Input: part model. Units: mm. Frame: model coordinates. Give positions to 0.01 mm unless a question says otherwise; leave off trailing zeros. Write each loop counter-clockwise with the first axis right and the second up, starting at its lowest first coordinate (ties: lowest second). Pieces come first, ordered by that corner, then holes. Notation, with made-up numbers: (76, -2) - (102, -2) arc R28 cw to (102, 21) - close; hole circle Ø7 at (8.25, 38.5). An arc over 180 degrees is marked (long way). Answer as CSV lines item,"result".
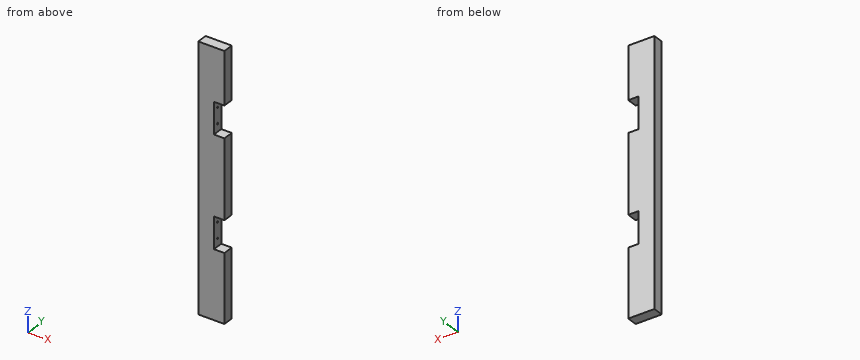
```python
from build123d import *

# Parameters (mm, degrees)
SKIZZE1_W                       = 50
SKIZZE1_H                       = 20
AUFSATZ_LINEAR_AUSTRAGEN1_DEPTH = 500
SKIZZE2_W                       = 20
SKIZZE2_H                       = 60
SCHNITT_LINEAR_AUSTRAGEN1_DEPTH = 502.023951523
SKIZZE3_R                       = 1.5
SCHNITT_LINEAR_AUSTRAGEN2_DEPTH = 20


with BuildPart() as part:
    # Skizze1 → Aufsatz-Linear austragen1 (new body)
    with BuildSketch(Plane.XY):
        Rectangle(SKIZZE1_W, SKIZZE1_H)
    extrude(amount=AUFSATZ_LINEAR_AUSTRAGEN1_DEPTH)

    # Skizze2 → Schnitt-Linear austragen1 (cut, through all)
    with BuildSketch(Plane(origin=(0, 10, 0), x_dir=(1, 0, 0), z_dir=(0, 1, 0))):
        with Locations((15, -370)):
            Rectangle(SKIZZE2_W, SKIZZE2_H)
        with Locations((15, -160)):
            Rectangle(SKIZZE2_W, SKIZZE2_H)
    extrude(amount=-SCHNITT_LINEAR_AUSTRAGEN1_DEPTH, mode=Mode.SUBTRACT)

    # Skizze3 → Schnitt-Linear austragen2 (cut)
    with BuildSketch(Plane(origin=(5, 0, 0), x_dir=(0, 0, -1), z_dir=(1, 0, 0))):
        with Locations((-385, 0)):
            Circle(SKIZZE3_R)
        with Locations((-355, 0)):
            Circle(SKIZZE3_R)
        with Locations((-175, 0)):
            Circle(SKIZZE3_R)
        with Locations((-145, 0)):
            Circle(SKIZZE3_R)
    extrude(amount=-SCHNITT_LINEAR_AUSTRAGEN2_DEPTH, mode=Mode.SUBTRACT)


solid = part.part
```
Item 1: Ray query, line 1 (Z direction, x = 13.5, y = -7.25); line 2 (Y direction, x = -4, z = 175); line 3 (X direction, y = -9, z = 132). Return the intervals inside material, ascending. Write a range as from..to.
The answers:
line 1,"0..130, 190..340, 400..500"
line 2,"-10..-1.5, 1.5..10"
line 3,"-25..5"
Item 2: Cut plane B-B on y = -4.75. Return the cut outline in (x, z), plus the area to 3 significant figures.
The answers:
outline,"(-25, 0) - (25, 0) - (25, 130) - (5, 130) - (5, 190) - (25, 190) - (25, 340) - (5, 340) - (5, 400) - (25, 400) - (25, 500) - (-25, 500) - close"
area,"22,600 mm²"
Item 3: Cut plane A-A on x = 11. Return the cut outline in (y, z), plus the area to 3 significant figures.
The answers:
outline,"(-10, 0) - (10, 0) - (10, 130) - (-10, 130) - close; (-10, 190) - (10, 190) - (10, 340) - (-10, 340) - close; (-10, 400) - (10, 400) - (10, 500) - (-10, 500) - close"
area,"7,600 mm²"
Item 4: Contact query for flat-ended pins moving along their axis: pin 1 (6 mm diameter, centred on y = 3.5, z = 362.5, fed in from +X); pin 2 (1.8 mm diameter, centred on y = 0, z = 385, fed in from +X). Output: stop coordinate, or through.
The answers:
pin 1,"x = 5"
pin 2,"x = -15"
